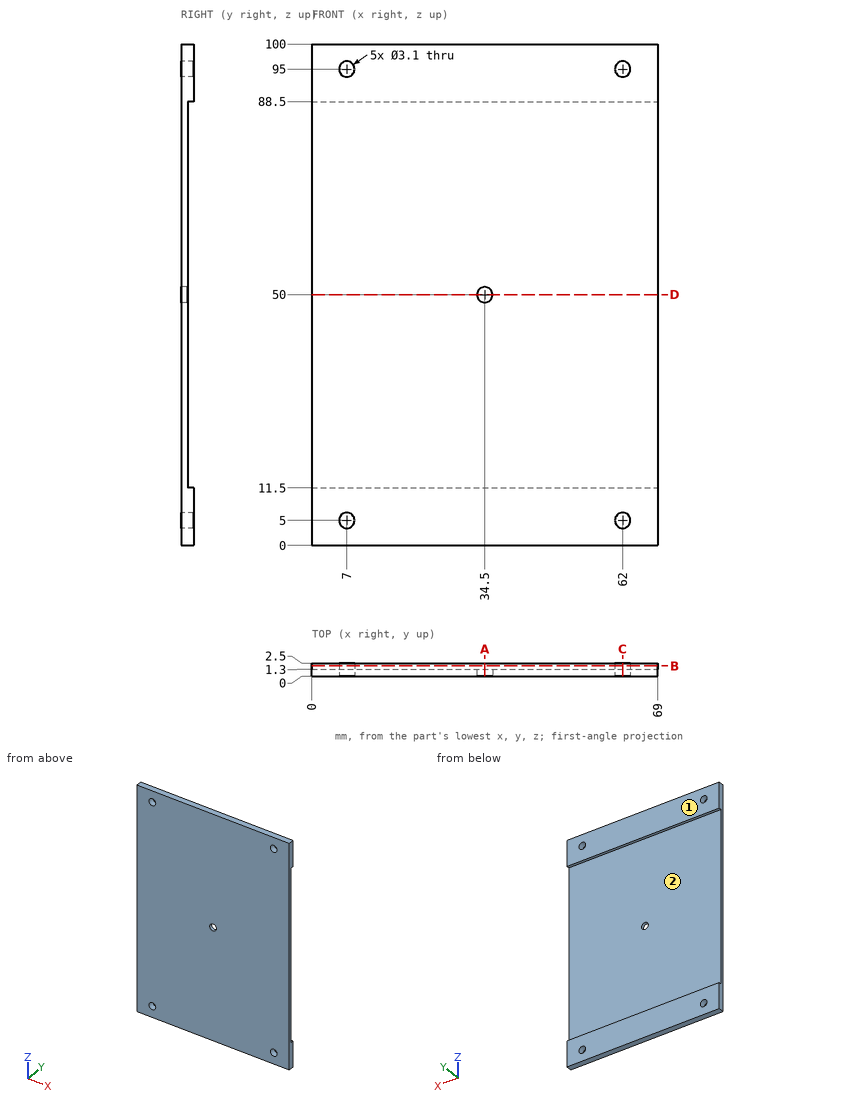
Drawing for the job (mm, zero at the part's lowest x, y, z). Coordinates: 2 decimals unless noted, no trailing zeros. Order: outer loops, then holes, each group sorted by start corner. A loop starts at its lowest first (then second) coordinate and runs counter-clockwise, first axis right, second up.
Item 1: Drill centre lines: L1, parallel to X at y = 0.6, z = 5; L2, parallel to Z at x = 62, y = 1.2; L3, parallel to Z at x = 33, y = 1.85. Where is each one in solid material? Low to high.
Check sheet entries:
L1: x = 0 to 5.45, 8.55 to 60.45, 63.55 to 69
L2: z = 0 to 3.45, 6.55 to 93.45, 96.55 to 100
L3: z = 0 to 11.5, 88.5 to 100
Item 2: Band-saw the part on D-D on z = 50. List the corners of the cut face in (x, y).
Check sheet entries:
outline: (0, 0) - (32.95, 0) - (32.95, 1.3) - (0, 1.3) - close; (36.05, 0) - (69, 0) - (69, 1.3) - (36.05, 1.3) - close
Item 3: Band-saw the part on B-B on y = 2. List the corners of the cut face in (x, z).
Check sheet entries:
outline: (0, 0) - (69, 0) - (69, 11.5) - (0, 11.5) - close; (0, 88.5) - (69, 88.5) - (69, 100) - (0, 100) - close; hole circle Ø3.1 at (7, 5); hole circle Ø3.1 at (7, 95); hole circle Ø3.1 at (62, 5); hole circle Ø3.1 at (62, 95)
Item 4: Two-plate mould, pull along Z, no slides. Class the marked faces 1 and 2: +Z half, -Z half, draft (parallel to the pull), parting line (faces both ways), or undercut.
Check sheet entries:
face 1: draft
face 2: undercut
Item 5: Band-saw the part on C-C on x = 62. List the corners of the cut face in (y, z).
Check sheet entries:
outline: (0, 0) - (2.5, 0) - (2.5, 3.45) - (0, 3.45) - close; (0, 6.55) - (2.5, 6.55) - (2.5, 11.5) - (1.3, 11.5) - (1.3, 88.5) - (2.5, 88.5) - (2.5, 93.45) - (0, 93.45) - close; (0, 96.55) - (2.5, 96.55) - (2.5, 100) - (0, 100) - close
Item 6: Band-saw the part on A-A on x = 34.5. List the corners of the cut face in (y, z).
Check sheet entries:
outline: (0, 0) - (2.5, 0) - (2.5, 11.5) - (1.3, 11.5) - (1.3, 48.45) - (0, 48.45) - close; (0, 51.55) - (1.3, 51.55) - (1.3, 88.5) - (2.5, 88.5) - (2.5, 100) - (0, 100) - close
